Geometry check sheet. Reference: the model listing, model coordinates, mm. Face numbers are marked on the shaded views. A direction names the side the tool comes from. Coordinates: 2 decimals unless noted, no trailing zeros. Loops run counter-clockwise (first coordinate to the right, second up) from the corner with the lowest first, then second, coordinate; pieces in that order, holes last. Notation, with made-up numbers: (11, 68) - (32, 68) arc R8 cw to (32, 75) - close; hole circle Ø9 at (35.5, 68.25). An arc over 180 degrees is marked (long way). Write each question's results on one line, items separated by ' | '. Start each with the question number.
(1) Sectioned sample at C-C (z = 3.25). Enter the section's corners in (x, y), plus the area to 3 significant figures.
(2) Go/stop test with flat-tipped pins: pin 1 Ø2.5 at (y, z) = (0.5, 8.5) entering from -X; pin 2 Ø3 at (x, z) = (1, 4.5) entering from -Y; pin 3 Ø2 at (x, z) = (-1.5, 3.5) entering from -Y; pin 4 Ø6 at (x, z) = (-2, 5) entering from +Y. Record where each tip stops, or that it passes through.
(3) Material ranges on probe 1 along Y at (x, z) = (-1.8, 0); probe 2 along X at (y, z) = (-9, -4); probe 3 along Y at (x, z) = (3.5, 0.25), recorded low to high.
(4) Sectioned sample at A-A (z = 0). Enter the section's corners in (x, y) (1 decimal), plus the area to 3 significant figures.
(5) Access from +Z, -Z, +X, -X, +Y, -Y to the whole of each face (thin tool, end or side, straight path). Record for the marked faces 4, 5, 6 and 7.
(6) Sectioned sample at B-B (y = -9). Enter the section's corners in (x, z), plus the area to 3 significant figures.
(7) Sectioned sample at D-D (y = 6.5). Enter the section's corners in (x, z).
(8) Mould release check, pull along Z, two halves, no side actions. Record for the marked faces 1, 2 and 3: pulls with the +Z half, pulls with the -Z half, needs draft (parallel to the pull), parting line crosses it, or undercut.
from build123d import *

# Parameters (mm, degrees)
OTHER_269_OUTLINE_R = 2.5
OTHER_269_DEPTH     = 8
EXTRUDE_START       = 4
SKETCH_1_R          = 7.8115
EXTRUDE_1_DEPTH     = 4
SKETCH_2_R          = 10.5
EXTRUDE_2_DEPTH     = 3
SKETCH_3_R          = 5
CUT_EXTRUDE_1_DEPTH = 18
SKETCH_4_R          = 1.25
CUT_EXTRUDE_2_DEPTH = 4


# Read off the part's stored shape, not the designer's step: звезда к рейки
with BuildPart() as part:
    # Other 269 outline → Other 269 (new body)
    with BuildSketch(Plane.YZ):
        with BuildLine():
            ThreePointArc((1.50889806, 10.517311997), (1.110614922, 10.566795138), (0.710747103, 10.601201043))
            ThreePointArc((0.710747103, 10.601201043), (0.052768817, 9.282126803), (-0.045978646, 7.811364683))
            ThreePointArc((-0.045978646, 7.811364683), (-0.816524091, 7.768707786), (-1.579100136, 7.650227121))
            ThreePointArc((-1.579100136, 7.650227121), (-1.98147837, 9.068318808), (-2.899329207, 10.221766733))
            ThreePointArc((-2.899329207, 10.221766733), (-3.283305565, 10.104975486), (-3.662597137, 9.973765949))
            ThreePointArc((-3.662597137, 9.973765949), (-3.727174383, 8.50110779), (-3.219171833, 7.117335524))
            ThreePointArc((-3.219171833, 7.117335524), (-3.90575, 6.764957442), (-4.554207455, 6.346552348))
            ThreePointArc((-4.554207455, 6.346552348), (-5.498588115, 7.478381595), (-6.806236115, 8.158785139))
            ThreePointArc((-6.806236115, 8.158785139), (-7.109512693, 7.895913771), (-7.402645059, 7.621776114))
            ThreePointArc((-7.402645059, 7.621776114), (-6.862655273, 6.250170009), (-5.835740964, 5.192654394))
            ThreePointArc((-5.835740964, 5.192654394), (-6.319636252, 4.591484498), (-6.741850931, 3.945501017))
            ThreePointArc((-6.741850931, 3.945501017), (-8.064942021, 4.595364266), (-9.536282966, 4.685075474))
            ThreePointArc((-9.536282966, 4.685075474), (-9.706420487, 4.321576832), (-9.862708399, 3.951911947))
            ThreePointArc((-9.862708399, 3.951911947), (-8.81152072, 2.918521053), (-7.443257466, 2.370116145))
            ThreePointArc((-7.443257466, 2.370116145), (-7.640799983, 1.624102173), (-7.763767133, 0.862236717))
            ThreePointArc((-7.763767133, 0.862236717), (-9.236794185, 0.917766707), (-10.617419857, 0.401273697))
            ThreePointArc((-10.617419857, 0.401273697), (-10.625, 0), (-10.617419857, -0.401273697))
            ThreePointArc((-10.617419857, -0.401273697), (-9.236794185, -0.917766707), (-7.763767133, -0.862236717))
            ThreePointArc((-7.763767133, -0.862236717), (-7.640799983, -1.624102173), (-7.443257466, -2.370116145))
            ThreePointArc((-7.443257466, -2.370116145), (-8.81152072, -2.918521053), (-9.862708399, -3.951911947))
            ThreePointArc((-9.862708399, -3.951911947), (-9.706420487, -4.321576832), (-9.536282966, -4.685075474))
            ThreePointArc((-9.536282966, -4.685075474), (-8.064942021, -4.595364266), (-6.741850931, -3.945501017))
            ThreePointArc((-6.741850931, -3.945501017), (-6.319636252, -4.591484498), (-5.835740964, -5.192654394))
            ThreePointArc((-5.835740964, -5.192654394), (-6.862655273, -6.250170009), (-7.402645059, -7.621776114))
            ThreePointArc((-7.402645059, -7.621776114), (-7.109512693, -7.895913771), (-6.806236115, -8.158785139))
            ThreePointArc((-6.806236115, -8.158785139), (-5.498588115, -7.478381595), (-4.554207455, -6.346552348))
            ThreePointArc((-4.554207455, -6.346552348), (-3.90575, -6.764957442), (-3.219171833, -7.117335524))
            ThreePointArc((-3.219171833, -7.117335524), (-3.727174383, -8.50110779), (-3.662597137, -9.973765949))
            ThreePointArc((-3.662597137, -9.973765949), (-3.283305565, -10.104975486), (-2.899329207, -10.221766733))
            ThreePointArc((-2.899329207, -10.221766733), (-1.98147837, -9.068318808), (-1.579100136, -7.650227121))
            ThreePointArc((-1.579100136, -7.650227121), (-0.816524091, -7.768707786), (-0.045978646, -7.811364683))
            ThreePointArc((-0.045978646, -7.811364683), (0.052768817, -9.282126803), (0.710747103, -10.601201043))
            ThreePointArc((0.710747103, -10.601201043), (1.110614922, -10.566795138), (1.50889806, -10.517311997))
            ThreePointArc((1.50889806, -10.517311997), (1.878246986, -9.090261316), (1.669047941, -7.631108125))
            ThreePointArc((1.669047941, -7.631108125), (2.413886252, -7.429177977), (3.135164666, -7.154737925))
            ThreePointArc((3.135164666, -7.154737925), (3.82358781, -8.458181767), (4.961196713, -9.395592168))
            ThreePointArc((4.961196713, -9.395592168), (5.3125, -9.201519915), (5.656223144, -8.99431847))
            ThreePointArc((5.656223144, -8.99431847), (5.413206375, -7.54041506), (4.628602467, -6.292501208))
            ThreePointArc((4.628602467, -6.292501208), (5.226913732, -5.805075804), (5.774209525, -5.26099198))
            ThreePointArc((5.774209525, -5.26099198), (6.933273734, -6.171740263), (8.353810339, -6.56540005))
            ThreePointArc((8.353810339, -6.56540005), (8.595805565, -6.245218306), (8.825535862, -5.916125569))
            ThreePointArc((8.825535862, -5.916125569), (8.012173204, -4.686762538), (6.787829577, -3.865863666))
            ThreePointArc((6.787829577, -3.865863666), (7.136160342, -3.177223287), (7.4148411, -2.457572728))
            ThreePointArc((7.4148411, -2.457572728), (8.844133643, -2.818148799), (10.301974266, -2.599990619))
            ThreePointArc((10.301974266, -2.599990619), (10.392818258, -2.209061715), (10.468833252, -1.81498081))
            ThreePointArc((10.468833252, -1.81498081), (9.225762498, -1.022726195), (7.773379287, -0.770783176))
            ThreePointArc((7.773379287, -0.770783176), (7.8115, 0), (7.773379287, 0.770783176))
            ThreePointArc((7.773379287, 0.770783176), (9.225762498, 1.022726195), (10.468833252, 1.81498081))
            ThreePointArc((10.468833252, 1.81498081), (10.392818258, 2.209061715), (10.301974266, 2.599990619))
            ThreePointArc((10.301974266, 2.599990619), (8.844133643, 2.818148799), (7.4148411, 2.457572728))
            ThreePointArc((7.4148411, 2.457572728), (7.136160342, 3.177223287), (6.787829577, 3.865863666))
            ThreePointArc((6.787829577, 3.865863666), (8.012173204, 4.686762538), (8.825535862, 5.916125569))
            ThreePointArc((8.825535862, 5.916125569), (8.595805565, 6.245218306), (8.353810339, 6.56540005))
            ThreePointArc((8.353810339, 6.56540005), (6.933273734, 6.171740263), (5.774209525, 5.26099198))
            ThreePointArc((5.774209525, 5.26099198), (5.226913732, 5.805075804), (4.628602467, 6.292501208))
            ThreePointArc((4.628602467, 6.292501208), (5.413206375, 7.54041506), (5.656223144, 8.99431847))
            ThreePointArc((5.656223144, 8.99431847), (5.3125, 9.201519915), (4.961196713, 9.395592168))
            ThreePointArc((4.961196713, 9.395592168), (3.82358781, 8.458181767), (3.135164666, 7.154737925))
            ThreePointArc((3.135164666, 7.154737925), (2.413886252, 7.429177977), (1.669047941, 7.631108125))
            ThreePointArc((1.669047941, 7.631108125), (1.878246986, 9.090261316), (1.50889806, 10.517311997))
        make_face()
        Circle(OTHER_269_OUTLINE_R, mode=Mode.SUBTRACT)
    extrude(amount=OTHER_269_DEPTH)

    # Эскиз1 → Бобышка-Вытянуть1 (add)
    with BuildSketch(Plane.ZY.offset(EXTRUDE_START)):
        Circle(SKETCH_1_R)
    extrude(amount=-EXTRUDE_1_DEPTH)

    # Эскиз2 → Бобышка-Вытянуть2 (add)
    with BuildSketch(Plane.ZY.offset(4)):
        Circle(SKETCH_2_R)
    extrude(amount=-EXTRUDE_2_DEPTH)

    # Эскиз3 → Вырез-Вытянуть1 (cut)
    with BuildSketch(Plane(origin=(8, 0, 0), x_dir=(0, 0, -1), z_dir=(1, 0, 0))):
        Circle(SKETCH_3_R)
    extrude(amount=-CUT_EXTRUDE_1_DEPTH, mode=Mode.SUBTRACT)

    # Эскиз4 → Вырез-Вытянуть2 (cut)
    with BuildSketch(Plane.ZY.offset(4)):
        with Locations((-7.5, 0)):
            Circle(SKETCH_4_R)
        with Locations((0, -7.474046633)):
            Circle(SKETCH_4_R)
        with Locations(Location((7.5, 0, 0), (0, 0, 279.848392372))):
            Circle(SKETCH_4_R)
        with Locations(Location((0, 7.474046633, 0), (0, 0, 11.094887122))):
            Circle(SKETCH_4_R)
    extrude(amount=-CUT_EXTRUDE_2_DEPTH, mode=Mode.SUBTRACT)


solid = part.part
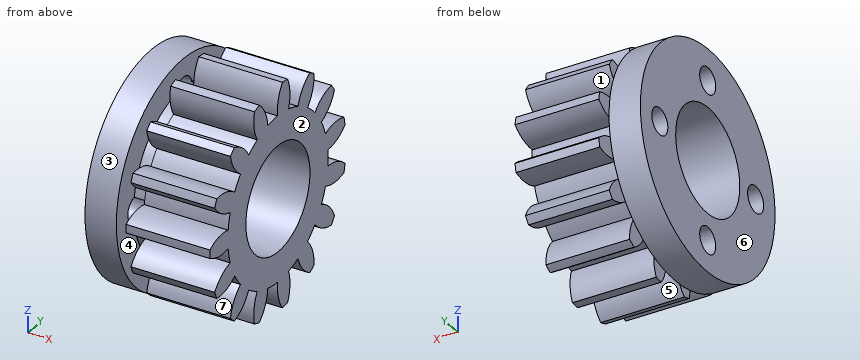
Outcome:
1) outline: (-4, -9.98) - (-1, -9.98) - (-1, -7.1) - (0, -7.1) - (0, -9.25) - (8, -9.25) - (8, -3.8) - (-4, -3.8) - close; (-4, 3.8) - (8, 3.8) - (8, 7.1) - (-1, 7.1) - (-1, 9.98) - (-4, 9.98) - close | area: 114 mm2
2) pin 1: stops at x = -4 | pin 2: stops at y = -9.86 | pin 3: stops at y = -10.2 | pin 4: stops at y = 10.31
3) probe 1: y = -10.5 to -8.72, -6.22 to -5, 5 to 6.22, 8.72 to 10.5 | probe 2: x = -4 to -1, 0 to 8 | probe 3: y = -10.62 to -4.99, 4.99 to 7.81
4) outline: (-4, -10.5) - (-1, -10.5) - (-1, -8.7) - (-4, -8.7) - close; (-4, -6.2) - (0, -6.2) - (0, -10.6) - (8, -10.6) - (8, -5) - (-4, -5) - close; (-4, 5) - (8, 5) - (8, 7.8) - (0, 7.8) - (0, 6.2) - (-4, 6.2) - close; (-4, 8.7) - (-1, 8.7) - (-1, 10.5) - (-4, 10.5) - close | area: 87.9 mm2
5) face 4: none | face 5: -Z, +X | face 6: +Z, -Z, -X, +Y, -Y | face 7: +X, -Y
6) outline: (-4, -5.41) - (-1, -5.41) - (-1, 5.41) - (-4, 5.41) - close; (0, -4.72) - (8, -4.72) - (8, -3.05) - (0, -3.05) - close; (0, -0.95) - (8, -0.95) - (8, 0.95) - (0, 0.95) - close; (0, 3.05) - (8, 3.05) - (8, 4.72) - (0, 4.72) - close | area: 74.3 mm2
7) outline: (-4, -8.25) - (-1, -8.25) - (-1, -4.33) - (0, -4.33) - (0, -5.91) - (8, -5.91) - (8, 5.91) - (0, 5.91) - (0, 4.33) - (-1, 4.33) - (-1, 8.25) - (-4, 8.25) - (-4, 0.78) - (0, 0.78) - (0, -0.78) - (-4, -0.78) - close
8) face 1: undercut | face 2: needs draft | face 3: parting line crosses it
